Job drawing, mm, ordinate dimensions from the low corner. One solid piece. A direction names the side the tool comes from. Give positions to 0.01 mm unless a question says otherwise; leave off trailing zeros. Write each loop counter-clockwise with the first axis right and the second up, starting at its lowest first coordinate (ties: lowest second). Pieces come first, ordered by that corner, then holes. Notation, with made-up numbers: (-8, -32.5) - (30, -32.5) arc R26 cw to (30, -12.5) - close; hole circle Ø6 at (-0.5, 76.5). An arc over 180 degrees is marked (long way). Answer in a Markdown table with one row per item. Add a question column.
1. Which spindle directions (+Z, -Z, +X, -X, +Y, -Y) get a long thin tool onto all of the face, cutting with end or side? Do the marked faces 1, 2 and 3. Say none if no direction does.
2. Band-saw the part on D-D on z = 3. Write the cut outline in (x, y), plus the area to 3 significant figures.
3. Band-saw the part on A-A on z = 1.2. Write the cut outline in (x, y), plus the area to 3 significant figures.
4. Band-saw the part on B-B on y = 9.5. Write the cut outline in (x, z).
5. Drop flat-ended pins along their axis: pin 1 Ø1.5 at (x, z) = (7.5, 2.5) entering from +Y; pin 2 Ø1.8 at (x, y) = (14.5, 18) entering from -Z; pin 3 Ø1.8 at (y, z) = (5, 2) entering from -X; pin 4 Ø1.8 at (y, z) = (9, 2) entering from +X. Give the stop position or say it passes through.
6. Pull direction Y, two halves, no side cores. Call the marked faces 4, 5, 6 and 7: released by +Y, released by -Y, zero draft, split by the parting line, or undercut.
7. Probe line 1 along Y through (x, z) = (8.5, 1.15); line 2 along Z through (x, y) = (8.5, 8); line 3 along Y through (x, z) = (10, 4.1). List the from-to ranges inside material, lowest first.
8. Band-saw the part on C-C on x = 2.5. Write the cut outline in (y, z).
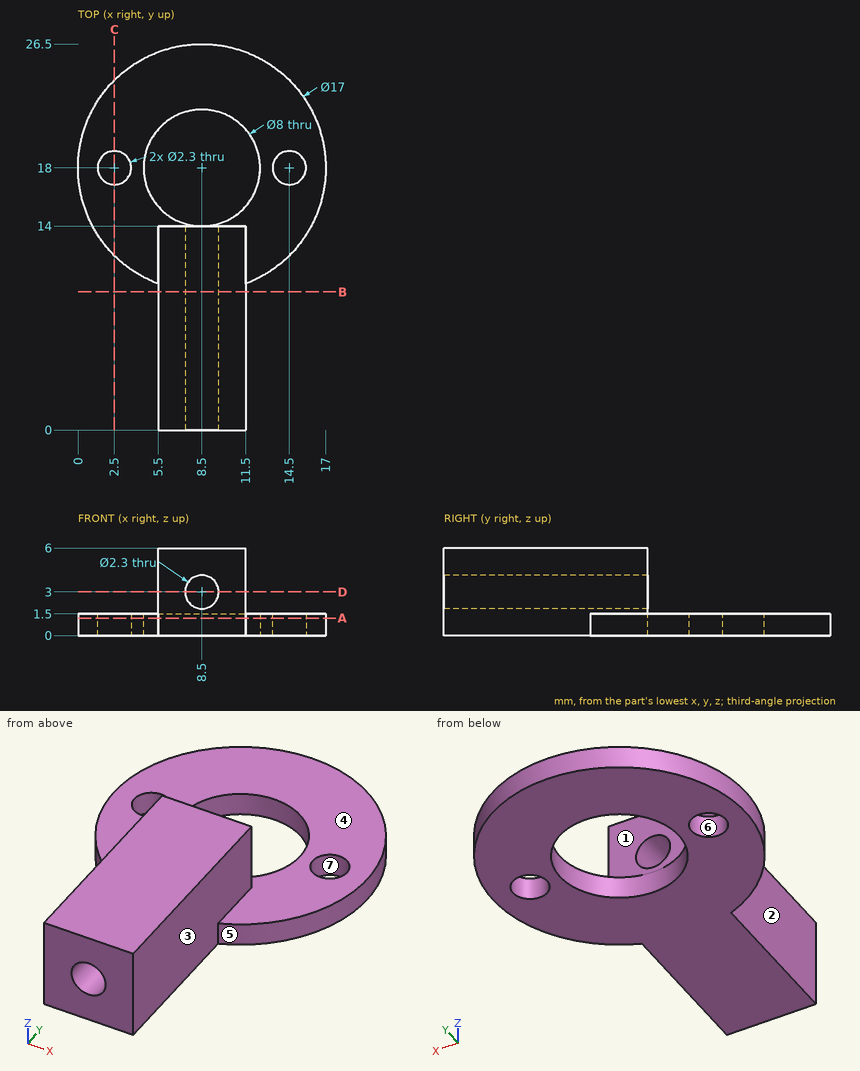
Values:
| question | item | result |
|---|---|---|
| 1 | face 1 | +Z, +X, -X, +Y |
| 1 | face 2 | +Z, -X, -Y |
| 1 | face 3 | +Z, +X, -Y |
| 2 | outline | (5.5, 0) - (7.35, 0) - (7.35, 14) - (5.5, 14) - close; (9.65, 0) - (11.5, 0) - (11.5, 14) - (9.65, 14) - close |
| 2 | area | 51.8 mm² |
| 3 | outline | (5.5, 0) - (11.5, 0) - (11.5, 10.05) arc R8.5 ccw (long way) to (5.5, 10.05) - close; hole circle Ø2.3 at (2.5, 18); hole circle Ø8 at (8.5, 18); hole circle Ø2.3 at (14.5, 18) |
| 3 | area | 226 mm² |
| 4 | outline | (5.5, 0) - (11.5, 0) - (11.5, 6) - (5.5, 6) - close; hole circle Ø2.3 at (8.5, 3) |
| 5 | pin 1 | stops at y = 14 |
| 5 | pin 2 | passes through |
| 5 | pin 3 | stops at x = 5.5 |
| 5 | pin 4 | stops at x = 11.5 |
| 6 | face 4 | zero draft |
| 6 | face 5 | split by the parting line |
| 6 | face 6 | undercut |
| 6 | face 7 | undercut |
| 7 | line 1 | y = 0 to 14, 22 to 26.5 |
| 7 | line 2 | z = 0 to 1.85, 4.15 to 6 |
| 7 | line 3 | y = 0 to 14 |
| 8 | outline | (11.98, 0) - (16.85, 0) - (16.85, 1.5) - (11.98, 1.5) - close; (19.15, 0) - (24.02, 0) - (24.02, 1.5) - (19.15, 1.5) - close |
